CAD build for the part. Positions are in the model's coordinates, mm. Coordinates: 2 decimals unless noted, no trailing zeros. Loops run counter-clockwise (first coordinate to the right, second up) from the corner with the lowest first, then second, coordinate; pieces in that order, holes last. Notation, with made-up numbers: M -11,23.5 L 40,23.5 A7 ccw 40,32.5 Z; hole C 74.25,10 d2. An arc over 180 degrees is marked long. Answer as a JSON object with one key per item and string values. Group by question number.
```python
from build123d import *

# Parameters (mm, degrees)
SKETCH1_W                  = 2.54
SKETCH1_H                  = 2.54
BOSS_EXTRUDE1_DEPTH        = 8.5
SKETCH2_W                  = 1
SKETCH2_H                  = 1
CUT_EXTRUDE1_DEPTH         = 8
CHAMFER1_SIZE              = 0.25
SKETCH3_R                  = 0.5
BOSS_EXTRUDE2_DEPTH        = 3
LPATTERN3_COUNT            = 20
LPATTERN3_PITCH            = 2.54
CHAMFER1_OF_LPATTERN3_SIZE = 0.25


with BuildPart() as part:
    # Sketch1 → Boss-Extrude1 (new body)
    with BuildSketch(Plane.XY):
        with Locations((1.27, 1.27)):
            Rectangle(SKETCH1_W, SKETCH1_H)
    boss_extrude1 = extrude(amount=BOSS_EXTRUDE1_DEPTH)

    # Sketch2 → Cut-Extrude1 (cut)
    with BuildSketch(Plane.XY.offset(8.5)):
        with Locations((1.27, 1.27)):
            Rectangle(SKETCH2_W, SKETCH2_H)
    cut_extrude1 = extrude(amount=-CUT_EXTRUDE1_DEPTH, mode=Mode.SUBTRACT)

    # Chamfer1
    chamfer1_edges = [part.edges().sort_by_distance(p)[0] for p in [
        (0.77, 1.27, 8.5),
        (1.27, 0.77, 8.5),
        (1.77, 1.27, 8.5),
        (1.27, 1.77, 8.5),
    ]]
    chamfer(chamfer1_edges, length=CHAMFER1_SIZE)

    # Sketch3 → Boss-Extrude2 (add)
    with BuildSketch(Plane(origin=(0, 0, 0), x_dir=(-1, 0, 0), z_dir=(0, 0, -1))):
        with Locations((-1.27, 1.27)):
            Circle(SKETCH3_R)
    boss_extrude2 = extrude(amount=BOSS_EXTRUDE2_DEPTH)

    # LPattern3: Boss-Extrude1, Cut-Extrude1, Boss-Extrude2 ×20
    with Locations(*[(i * LPATTERN3_PITCH, 0, 0) for i in range(1, LPATTERN3_COUNT)]):
        add(boss_extrude1)
        add(cut_extrude1, mode=Mode.SUBTRACT)
        add(boss_extrude2)

    # Chamfer1 of LPattern3
    chamfer1_of_lpattern3_edges = [part.edges().sort_by_distance(p)[0] for p in [
        (3.31, 1.27, 8.5),
        (3.81, 0.77, 8.5),
        (4.31, 1.27, 8.5),
        (3.81, 1.77, 8.5),
        (5.85, 1.27, 8.5),
        (6.35, 0.77, 8.5),
        (6.85, 1.27, 8.5),
        (6.35, 1.77, 8.5),
        (8.39, 1.27, 8.5),
        (8.89, 0.77, 8.5),
        (9.39, 1.27, 8.5),
        (8.89, 1.77, 8.5),
        (10.93, 1.27, 8.5),
        (11.43, 0.77, 8.5),
        (11.93, 1.27, 8.5),
        (11.43, 1.77, 8.5),
        (13.47, 1.27, 8.5),
        (13.97, 0.77, 8.5),
        (14.47, 1.27, 8.5),
        (13.97, 1.77, 8.5),
        (16.01, 1.27, 8.5),
        (16.51, 0.77, 8.5),
        (17.01, 1.27, 8.5),
        (16.51, 1.77, 8.5),
        (18.55, 1.27, 8.5),
        (19.05, 0.77, 8.5),
        (19.55, 1.27, 8.5),
        (19.05, 1.77, 8.5),
        (21.09, 1.27, 8.5),
        (21.59, 0.77, 8.5),
        (22.09, 1.27, 8.5),
        (21.59, 1.77, 8.5),
        (23.63, 1.27, 8.5),
        (24.13, 0.77, 8.5),
        (24.63, 1.27, 8.5),
        (24.13, 1.77, 8.5),
        (26.17, 1.27, 8.5),
        (26.67, 0.77, 8.5),
        (27.17, 1.27, 8.5),
        (26.67, 1.77, 8.5),
        (28.71, 1.27, 8.5),
        (29.21, 0.77, 8.5),
        (29.71, 1.27, 8.5),
        (29.21, 1.77, 8.5),
        (31.25, 1.27, 8.5),
        (31.75, 0.77, 8.5),
        (32.25, 1.27, 8.5),
        (31.75, 1.77, 8.5),
        (33.79, 1.27, 8.5),
        (34.29, 0.77, 8.5),
        (34.79, 1.27, 8.5),
        (34.29, 1.77, 8.5),
        (36.33, 1.27, 8.5),
        (36.83, 0.77, 8.5),
        (37.33, 1.27, 8.5),
        (36.83, 1.77, 8.5),
        (38.87, 1.27, 8.5),
        (39.37, 0.77, 8.5),
        (39.87, 1.27, 8.5),
        (39.37, 1.77, 8.5),
        (41.41, 1.27, 8.5),
        (41.91, 0.77, 8.5),
        (42.41, 1.27, 8.5),
        (41.91, 1.77, 8.5),
        (43.95, 1.27, 8.5),
        (44.45, 0.77, 8.5),
        (44.95, 1.27, 8.5),
        (44.45, 1.77, 8.5),
        (46.49, 1.27, 8.5),
        (46.99, 0.77, 8.5),
        (47.49, 1.27, 8.5),
        (46.99, 1.77, 8.5),
        (49.03, 1.27, 8.5),
        (49.53, 0.77, 8.5),
        (50.03, 1.27, 8.5),
        (49.53, 1.77, 8.5),
    ]]
    chamfer(chamfer1_of_lpattern3_edges, length=CHAMFER1_OF_LPATTERN3_SIZE)


solid = part.part
```
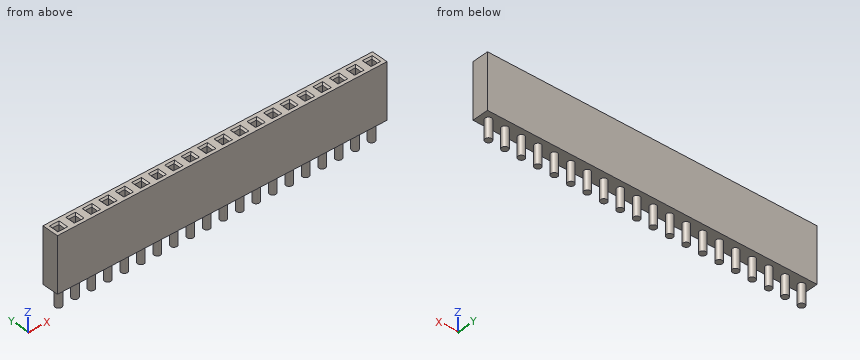
Item 1: Pin check, flat tip, straight feed: pin 1 (1 mm diameter, centred on x = 6.5, y = 2, fed in from -Z). Stop position of the tip, or through.
Item 2: Slice it at B-B, the plane z = 1.75. Count the separate pieces of the cut face and the enclosed holes in it, then the cut area to 3 significant figures.
Item 3: Drill centre lines: L1, parallel to Z at x = 6.5, y = 2.2; L2, parallel to Z at x = 39.5, y = 1.05; L3, parallel to Y at x = 26.5, z = 4. Where is each one in solid material? Low to high. Write a range as from..to.
Item 4: Slice it at A-A, the plane x = 6.35. Write the cut outline in (y, z), then the cut area to 3 significant figures.
Computed:
{
 "1": {"pin 1": "z = -3"},
 "2": {"separate pieces": "1", "enclosed holes": "20", "area": "109 mm2"},
 "3": {"L1": "0..8.5", "L2": "-3..0.5", "L3": "0..0.77, 1.77..2.54"},
 "4": {"outline": "M 0,0 L 0.77,0 L 0.77,-3 L 1.77,-3 L 1.77,0 L 2.54,0 L 2.54,8.5 L 2.02,8.5 L 1.77,8.25 L 1.77,0.5 L 0.77,0.5 L 0.77,8.25 L 0.52,8.5 L 0,8.5 Z", "area": "16.5 mm2"}
}
